Source: CAD feature listing. Evaluate the final solid. Frame: model axes, mm. Face numbers are marked on the shaded views. A direction names the side the tool comes from. Coordinates: 2 decimals unless noted, no trailing zeros. Loops run counter-clockwise (first coordinate to the right, second up) from the corner with the lowest first, then second, coordinate; pieces in that order, holes last. Notation, with made-up numbers: (66, -32) -> (71, -32) arc R28 ccw to (71, 0) -> close; hole circle Ø2 at (-9.75, 4). An arc over 180 degrees is marked (long way). Answer as CSV lines item,"result".
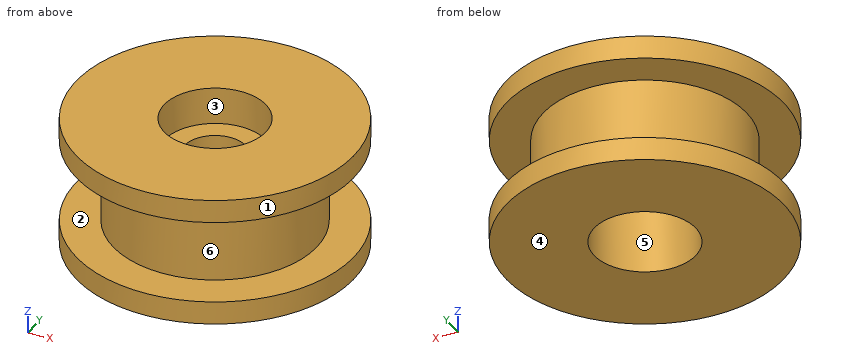
from build123d import *

# Parameters (mm, degrees)
SKETCH2_R          = 3
CUT_EXTRUDE1_DEPTH = 2
SKETCH3_R          = 2.75
CUT_EXTRUDE2_DEPTH = 2


with BuildPart() as part:
    # Sketch1 → Revolve1 (revolve)
    with BuildSketch(Plane(origin=(0, 0, 0), x_dir=(1, 0, 0), z_dir=(0, 1, 0))):
        Polygon((1.65, 0), (7.5, 0), (7.5, 1.25), (5.5, 1.25), (5.5, 5.75), (7.5, 5.75), (7.5, 7), (3, 7), (3, 9), (2.75, 9), (2.75, 3), (1.65, 3), align=None)
    revolve(axis=Axis((0, 0, 0), (0, 0, -1)))

    # Sketch2 → Cut-Extrude1 (cut)
    with BuildSketch(Plane(origin=(0, 0, -9), x_dir=(-1, 0, 0), z_dir=(0, 0, -1))):
        Circle(SKETCH2_R)
    extrude(amount=-CUT_EXTRUDE1_DEPTH, mode=Mode.SUBTRACT)

    # Sketch3 → Cut-Extrude2 (cut)
    with BuildSketch(Plane.XY):
        Circle(SKETCH3_R)
    extrude(amount=-CUT_EXTRUDE2_DEPTH, mode=Mode.SUBTRACT)


solid = part.part
(1) Material intervals for L1, parallel to Z at x = 4.75, y = 4.5; L2, parallel to Y at x = 0, z = -2.15; L3, parallel to Y at x = 0, z = -0.75, sorted ascending. Write a range as [from, to].
Computed values:
L1,"[-7, -5.75], [-1.25, 0]"
L2,"[-5.5, -1.65], [1.65, 5.5]"
L3,"[-7.5, -2.75], [2.75, 7.5]"
(2) Access query for the marked faces 1 and 2. Directions: +Z, -Z, +X, -X, +Y, -Y. A direction counts if a zero-diameter tool reaches every point of the face in a straight line with its end or side. Return the directions, or none.
Computed values:
face 1,"+Z, -Z"
face 2,"none"
(3) Pin query (flat end, axial travel): pin 1 Ø3.5 at (x, y) = (0, 0) entering from -Z; pin 2 Ø1.5 at (x, z) = (-4.5, -4) entering from +Y. Return the tip coordinate at first contact, or that it passes through.
Computed values:
pin 1,"z = -3"
pin 2,"y = 4.02"
(4) Cut plane D-D (y = -4). Return the cut outline in (x, z), then the cut area to 3 significant figures.
Computed values:
outline,"(-6.34, -7) -> (6.34, -7) -> (6.34, -5.75) -> (3.77, -5.75) -> (3.77, -1.25) -> (6.34, -1.25) -> (6.34, 0) -> (-6.34, 0) -> (-6.34, -1.25) -> (-3.77, -1.25) -> (-3.77, -5.75) -> (-6.34, -5.75) -> close"
area,"65.7 mm^2"
(5) Cut plane A-A (y = 0). Return the cut outline in (x, z), then the cut area to 3 significant figures.
Computed values:
outline,"(-7.5, -7) -> (-2.75, -7) -> (-2.75, -3) -> (-1.65, -3) -> (-1.65, -2) -> (-2.75, -2) -> (-2.75, 0) -> (-7.5, 0) -> (-7.5, -1.25) -> (-5.5, -1.25) -> (-5.5, -5.75) -> (-7.5, -5.75) -> close; (1.65, -3) -> (2.75, -3) -> (2.75, -7) -> (7.5, -7) -> (7.5, -5.75) -> (5.5, -5.75) -> (5.5, -1.25) -> (7.5, -1.25) -> (7.5, 0) -> (2.75, 0) -> (2.75, -2) -> (1.65, -2) -> close"
area,"50.7 mm^2"
(6) Cut plane C-C (z = -1). Return the cut outline in (x, y), then the cut area to 3 significant figures.
Computed values:
outline,"circle Ø15 at (0, 0); hole circle Ø5.5 at (0, 0)"
area,"153 mm^2"
(7) Draft query along X for the marked faces 3, 4, 5 and 6. Return one class per face: released by +X, released by -X, zero draft, split by the parting line, or undercut.
Computed values:
face 3,"undercut"
face 4,"zero draft"
face 5,"undercut"
face 6,"split by the parting line"
